from build123d import *

# Parameters (mm, degrees)
EXTRUDE_1_DEPTH     = 1200
CUT_EXTRUDE_1_DEPTH = 38.43114855


with BuildPart() as part:
    # Эскиз2 → Бобышка-Вытянуть1 (new body)
    with BuildSketch(Plane(origin=(0, 0, 0), x_dir=(0, 0, -1), z_dir=(1, 0, 0))):
        Polygon((0, 20), (0, 0), (-400, 0), (-599.238939618, -17.43114855), (-599.238939618, 2.56885145), (-400, 20), align=None)
    extrude(amount=-EXTRUDE_1_DEPTH)

    # Эскиз3 → Вырез-Вытянуть1 (cut, through all)
    with BuildSketch(Plane(origin=(0, 20, 0), x_dir=(1, 0, 0), z_dir=(0, 1, 0))):
        with BuildLine():
            Line((-822.385668675, -599.238939618), (-377.614331325, -599.238939618))
            Line((-377.614331325, -599.238939618), (-426.451140145, -514.835069456))
            ThreePointArc((-426.451140145, -514.835069456), (-444.74923451, -496.562846761), (-469.728809412, -489.875902964))
            Line((-469.728809412, -489.875902964), (-730.271190588, -489.875902964))
            ThreePointArc((-730.271190588, -489.875902964), (-755.25076549, -496.562846761), (-773.548859855, -514.835069456))
            Line((-773.548859855, -514.835069456), (-822.385668675, -599.238939618))
        make_face()
    extrude(amount=-CUT_EXTRUDE_1_DEPTH, mode=Mode.SUBTRACT)


solid = part.part
Geometry: final body of the model. Coordinates: model frame, mm. A direction names the side the tool comes from. Give positions to 0.01 mm unless a question says otherwise; leave off trailing zeros. Write each loop counter-clockwise with the first axis right and the second up, starting at its lowest first coordinate (ties: lowest second). Pieces come first, ordered by that corner, then holes.
(1) Cut plane A-A, the plane z = 527.5. Return loops of the section in (x, y).
(2) Ray query, line 1 (X direction, y = 0, z = 569.5); line 2 (Y direction, x = -570, z = 154); line 3 (Z direction, x = -621.5, y = 10.5). Return the intervals inside material, ascending.
(3) Access query for faces 1 (the flat face through (-1200, 6, 295)), 2 (the flat face through (-592, 0, 197)), 3 (the flat face through (-401.69, -3.55, 557.63)). Directions: +Z, -Z, +X, -X, +Y, -Y. A direction counts if a zero-diameter tool reaches every point of the face in a straight line with its end or side. Return the directions, or none.
(4) Mould query, pull axis X, two halves, no side actions, for faces 4 (the flat face through (0, 6, 295)), 5 (the flat face through (-591.6, -6.657, 476.087)), 6 (the cylindrical face through (-444.43, 1.2, 496.75)). Classes: released by +X, released by -X, zero draft, split by the parting line, or undercut.
(5) Cut plane B-B, the plane x = -229.5. Return loops of the section in (y, z), then the cut area to 3 significant figures.
(6) First-contact query: P1, Ø5, axis at x = -882.5, z = 305, coming from the -Y side; P2, Ø16, axis at x = -664, y = -0.5, coming from the +Z side. Flat tips, straight axial feed; report the tip coordinate or a pass-through.
(7) Cut plane C-C, the plane z = 87.5. Return loops of the section in (x, y), then the cut area to 3 significant figures.
Values follow:
1. outline: (-1200, -11.15) - (-780.88, -11.15) - (-780.88, 8.85) - (-1200, 8.85) - close; (-419.12, -11.15) - (0, -11.15) - (0, 8.85) - (-419.12, 8.85) - close
2. line 1: x = -1200 to -805.18, -394.82 to 0
2. line 2: y = 0 to 20
2. line 3: z = 0 to 489.88
3. face 1: +Z, -Z, -X, +Y, -Y
3. face 2: -Z, +X, -X, -Y
3. face 3: +Z, +Y, -Y
4. face 4: released by +X
4. face 5: zero draft
4. face 6: undercut
5. outline: (-17.43, 599.24) - (0, 400) - (0, 0) - (20, 0) - (20, 400) - (2.57, 599.24) - close
5. area: 12,000 mm2
6. P1: stops at y = 0
6. P2: stops at z = 489.88
7. outline: (-1200, 0) - (0, 0) - (0, 20) - (-1200, 20) - close
7. area: 24,000 mm2
